```python
from build123d import *

# Parameters (mm, degrees)
SKETCH1_R           = 1.6
SKETCH1_R_2         = 1.961338098
SKETCH1_W           = 40.698202598
SKETCH1_H           = 20.498202598
BOSS_EXTRUDE1_DEPTH = 3.5


with BuildPart() as part:
    # Sketch1 → Boss-Extrude1 (new body)
    with BuildSketch(Plane.XY):
        with BuildLine():
            ThreePointArc((-50.044200549, -24.884800983), (-49.571119709, -26.026919161), (-48.429001531, -26.5))
            Line((-48.429001531, -26.5), (45.955799451, -26.5))
            ThreePointArc((45.955799451, -26.5), (48.784226576, -25.328427125), (49.955799451, -22.5))
            Line((49.955799451, -22.5), (49.955799451, 22.5))
            ThreePointArc((49.955799451, 22.5), (48.784226576, 25.328427125), (45.955799451, 26.5))
            Line((45.955799451, 26.5), (-48.429001531, 26.5))
            ThreePointArc((-48.429001531, 26.5), (-49.571119709, 26.026919161), (-50.044200549, 24.884800983))
            Line((-50.044200549, 24.884800983), (-50.044200549, -24.884800983))
        make_face()
        with Locations((-44.044200549, -20.5)):
            Circle(SKETCH1_R, mode=Mode.SUBTRACT)
        with Locations((-14.462088638, -5)):
            Circle(SKETCH1_R_2, mode=Mode.SUBTRACT)
        with BuildLine():
            ThreePointArc((12.196121371, -14.531845007), (-0.008459876, -18.999966384), (-12.229764581, -14.57779233))
            ThreePointArc((-12.229764581, -14.57779233), (-12.355671334, -13.169194626), (-10.94707363, -13.043287874))
            ThreePointArc((-10.94707363, -13.043287874), (-0.012222052, -16.999969923), (10.907666432, -13.002177111))
            ThreePointArc((10.907666432, -13.002177111), (12.31672785, -13.122783589), (12.196121371, -14.531845007))
        make_face(mode=Mode.SUBTRACT)
        with Locations((43.955799451, -20.5)):
            Circle(SKETCH1_R, mode=Mode.SUBTRACT)
        with Locations((10, 0)):
            Rectangle(SKETCH1_W, SKETCH1_H, mode=Mode.SUBTRACT)
        with Locations((34.462088638, -5)):
            Circle(SKETCH1_R_2, mode=Mode.SUBTRACT)
        with Locations((-14.462088638, 5)):
            Circle(SKETCH1_R_2, mode=Mode.SUBTRACT)
        with Locations((-44.044200549, 20.5)):
            Circle(SKETCH1_R, mode=Mode.SUBTRACT)
        with Locations((34.462088638, 5)):
            Circle(SKETCH1_R_2, mode=Mode.SUBTRACT)
        with BuildLine():
            ThreePointArc((-10.94707363, 13.043287874), (-12.355671334, 13.169194626), (-12.229764581, 14.57779233))
            ThreePointArc((-12.229764581, 14.57779233), (-0.008459876, 18.999966384), (12.196121371, 14.531845007))
            ThreePointArc((12.196121371, 14.531845007), (12.31672785, 13.122783589), (10.907666432, 13.002177111))
            ThreePointArc((10.907666432, 13.002177111), (-0.012222052, 16.999969923), (-10.94707363, 13.043287874))
        make_face(mode=Mode.SUBTRACT)
        with Locations((43.955799451, 20.5)):
            Circle(SKETCH1_R, mode=Mode.SUBTRACT)
    extrude(amount=BOSS_EXTRUDE1_DEPTH)


solid = part.part
```
Source: CAD feature listing. Evaluate the final solid. Frame: model axes, mm. A direction names the side the tool comes from. Coordinates: 2 decimals unless noted, no trailing zeros. Write each loop counter-clockwise with the first axis right and the second up, starting at its lowest first coordinate (ties: lowest second). Pieces come first, ordered by that corner, then holes. Notation, with made-up numbers: (84, 41) -> (97, 41) arc R28 ccw to (97, 68) -> close; hole circle Ø8 at (-21, 11.25). An arc over 180 degrees is marked (long way). Return JSON: item names as keys, results as strings. Group by question number.
1) Section query A-A, the plane y = -9. Return loops of the section in (x, z), plus the area to 3 significant figures.
2) Section query B-B, the plane y = 20.5. Return loops of the section in (x, z), plus the area to 3 significant figures.
3) Contact query for a flat-ended pin moving along its axis: P1, Ø2.5, axis at x = 34.46, y = -5, coming from the +Z side. Output: stop coordinate, or through.
4) Mould query, pull axis Y, two halves, no side actions, for faces 1 (the face through (-1, 26.5, 2)), 2 (the face through (-12, 0, 0)), 3 (the face through (-12.37, -13.186, 1.726)). Classes: +Y half, -Y half, draft (parallel to the pull), parting line (faces both ways), or undercut.
5) Section query D-D, the plane x = 34.5. Return loops of the section in (y, z).
6) Section query C-C, the plane x = 17. Return loops of the section in (y, z), plus the area to 3 significant figures.
7) Set-up query: faces 4 (the face through (0, -19, 2)), 5 (the face through (-12, 0, 3.5)). Return all of +Z, -Z, +X, -X, +Y, -Y with unobstructed straight access to the full face (end or side cutting, diameter ignored); none if empty.
8) Ray query, line 1 along Y through (x, z) = (8.5, 2.75); line 2 along Y through (x, z) = (28.5, 0.4); line 3 along Y through (x, z) = (7.5, 2.25). Return the intervals inside material, ascending.
From the geometry:
{
 "1": {"outline": "(-50.04, 0) -> (-10.35, 0) -> (-10.35, 3.5) -> (-50.04, 3.5) -> close; (30.35, 0) -> (49.96, 0) -> (49.96, 3.5) -> (30.35, 3.5) -> close", "area": "208 mm²"},
 "2": {"outline": "(-50.04, 0) -> (-45.64, 0) -> (-45.64, 3.5) -> (-50.04, 3.5) -> close; (-42.44, 0) -> (42.36, 0) -> (42.36, 3.5) -> (-42.44, 3.5) -> close; (45.56, 0) -> (49.96, 0) -> (49.96, 3.5) -> (45.56, 3.5) -> close", "area": "328 mm²"},
 "3": {"P1": "through"},
 "4": {"face 1": "+Y half", "face 2": "draft", "face 3": "undercut"},
 "5": {"outline": "(-26.5, 0) -> (-6.96, 0) -> (-6.96, 3.5) -> (-26.5, 3.5) -> close; (-3.04, 0) -> (3.04, 0) -> (3.04, 3.5) -> (-3.04, 3.5) -> close; (6.96, 0) -> (26.5, 0) -> (26.5, 3.5) -> (6.96, 3.5) -> close"},
 "6": {"outline": "(-26.5, 0) -> (-10.25, 0) -> (-10.25, 3.5) -> (-26.5, 3.5) -> close; (10.25, 0) -> (26.5, 0) -> (26.5, 3.5) -> (10.25, 3.5) -> close", "area": "114 mm²"},
 "7": {"face 4": "+Z, -Z", "face 5": "+Z, +X, -X, +Y, -Y"},
 "8": {"line 1": "-26.5 to -16.97, -14.7 to -10.25, 10.25 to 14.7, 16.97 to 26.5", "line 2": "-26.5 to -10.25, 10.25 to 26.5", "line 3": "-26.5 to -17.44, -15.23 to -10.25, 10.25 to 15.23, 17.44 to 26.5"}
}
